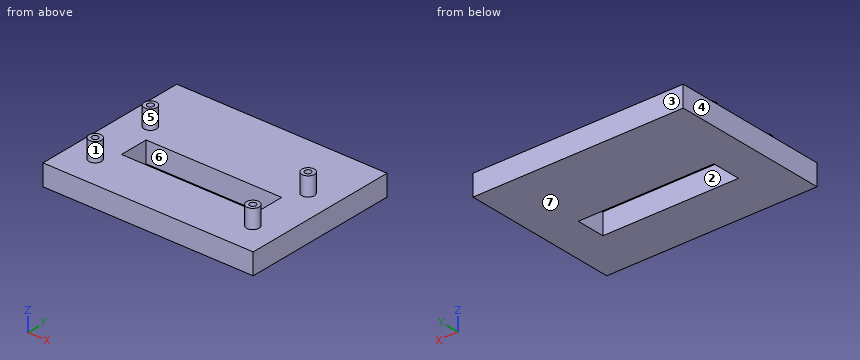
```python
from build123d import *

# Parameters (mm, degrees)
SKETCH_W      = 100
SKETCH_H      = 75
PAD_DEPTH     = 10
SKETCH001_R   = 3
SKETCH001_R_2 = 1.5
PAD001_DEPTH  = 8.9
POCKET_DEPTH  = 10


with BuildPart() as part:
    # Sketch → Pad (new body)
    with BuildSketch(Plane.XY):
        with Locations((50, 37.5)):
            Rectangle(SKETCH_W, SKETCH_H)
    extrude(amount=PAD_DEPTH)

    # Sketch001 → Pad001 (new body)
    with BuildSketch(Plane.XY.offset(10)):
        with Locations((12.5, 14.5)):
            Circle(SKETCH001_R)
        with Locations((12.5, 14.5)):
            Circle(SKETCH001_R_2, mode=Mode.SUBTRACT)
        with Locations((12.5, 45.5)):
            Circle(SKETCH001_R)
        with Locations((12.5, 45.5)):
            Circle(SKETCH001_R_2, mode=Mode.SUBTRACT)
        with Locations((87.5, 45.5)):
            Circle(SKETCH001_R)
        with Locations((87.5, 45.5)):
            Circle(SKETCH001_R_2, mode=Mode.SUBTRACT)
        with Locations((87.5, 14.5)):
            Circle(SKETCH001_R)
        with Locations((87.5, 14.5)):
            Circle(SKETCH001_R_2, mode=Mode.SUBTRACT)
    extrude(amount=PAD001_DEPTH)

    # Sketch002 → Pocket (cut)
    with BuildSketch(Plane.XY.offset(10)):
        Polygon((82.25, 23.1), (82.25, 36.9), (17.75, 36.9), (17.75, 30), (17.75, 23.1), (50, 23.1), align=None)
    extrude(amount=-POCKET_DEPTH, mode=Mode.SUBTRACT)


solid = part.part
```
The listing builds one solid part. Answer for the finished solid, in the listing's coordinates (mm). Face numbers are marked on the shaded views. A direction names the side the tool comes from. Coordinates: 2 decimals unless noted, no trailing zeros. Order: outer loops, then holes, each group sorted by start corner. A loop starts at its lowest first (then second) coordinate and runs counter-clockwise, first axis right, second up. Notation, with made-up numbers: M 50,44 L 103,44 A21 cw 103,68 Z; hole C 50.25,39 d8. An arc over 180 degrees is marked long. Answer as a JSON object with one key per item and string values. Group by question number.
1. Section D-D on y = 45.5 is taken. Write down the section's boundary in (x, z), then the cut area to 3 significant figures.
2. Determine the mould class of the marked faces 1, 2, 3 and 4 for opening direction X: released by +X, released by -X, zero draft, split by the parting line, or undercut.
3. Section A-A on z = 14.5 is taken. Write down the section's boundary in (x, y), then the cut area to 3 significant figures.
4. Section C-C on y = 34 is taken. Write down the section's boundary in (x, z).
5. A tool of negligible diameter and unlimited length cuts with its end or side. For the marked faces 5, 6 and 7, from which of +Z, -Z, +X, -X, +Y, -Y can it reach the whole face along a straight path? Write none if from no direction.
6. Section B-B on x = 70.5 is taken. Write down the section's boundary in (y, z).
7. Flat-ended cylindrical pins translate along their axes: P1, Ø2, axis at x = 81, y = 17.5, coming from the +Z side; P2, Ø1.5, axis at y = 16, z = 14, coming from the +X side; P3, Ø4, axis at x = 19, z = 13, coming from the -Y side. Find the tip coordinate at first contact, or state that the pin passes through.
8. Straight lines are drawn through the part: line 1 (Y direction, x = 87.5, z = 12.5); line 2 (Y direction, x = 65, z = 3); line 3 (Z direction, x = 90, y = 30). For each, find the intervals that lie inside material, in ascending order.
Values follow:
{
 "1": {"outline": "M 0,0 L 100,0 L 100,10 L 90.5,10 L 90.5,18.9 L 89,18.9 L 89,10 L 86,10 L 86,18.9 L 84.5,18.9 L 84.5,10 L 15.5,10 L 15.5,18.9 L 14,18.9 L 14,10 L 11,10 L 11,18.9 L 9.5,18.9 L 9.5,10 L 0,10 Z", "area": "1,050 mm2"},
 "2": {"face 1": "undercut", "face 2": "undercut", "face 3": "zero draft", "face 4": "released by -X"},
 "3": {"outline": "C 12.5,14.5 d6; C 12.5,45.5 d6; C 87.5,14.5 d6; C 87.5,45.5 d6; hole C 12.5,14.5 d3; hole C 12.5,45.5 d3; hole C 87.5,14.5 d3; hole C 87.5,45.5 d3", "area": "84.8 mm2"},
 "4": {"outline": "M 0,0 L 17.75,0 L 17.75,10 L 0,10 Z; M 82.25,0 L 100,0 L 100,10 L 82.25,10 Z"},
 "5": {"face 5": "+Z", "face 6": "+Z, -Z", "face 7": "-Z, +X, -X, +Y, -Y"},
 "6": {"outline": "M 0,0 L 23.1,0 L 23.1,10 L 0,10 Z; M 36.9,0 L 75,0 L 75,10 L 36.9,10 Z"},
 "7": {"P1": "z = 10", "P2": "x = 90.4", "P3": "through"},
 "8": {"line 1": "11.5 to 13, 16 to 17.5, 42.5 to 44, 47 to 48.5", "line 2": "0 to 23.1, 36.9 to 75", "line 3": "0 to 10"}
}
